from build123d import *

# Parameters (mm, degrees)
F2_R     = 1.5875
F3_DEPTH = 8.891
F4_SIZE  = 0.508
F5_SIZE  = 0.508


with BuildPart() as f1:
    # F0 (on Front) → F1 (revolve)
    with BuildSketch(Plane.XZ):
        Polygon((0.508, 6.35), (0, 6.35), (-0.508, 6.35), (-0.508, 10.16), (-2.0955, 10.16), (-4.445, 6.35), (-4.445, 0), (4.445, 0), (4.445, 6.35), (2.0955, 10.16), (0.508, 10.16), align=None)
    revolve(axis=Axis((0, 0, 0), (-1, 0, 0)))

    # F2 (on face) → F3 (cut, through all)
    with BuildSketch(Plane.YZ.offset(4.445)):
        Circle(F2_R)
    extrude(amount=-F3_DEPTH, mode=Mode.SUBTRACT)

    # F4
    f4_edges = [f1.edges().sort_by_distance(p)[0] for p in [
        (-4.445, -1.5875, 0),
        (4.445, -1.5875, 0),
    ]]
    chamfer(f4_edges, length=F4_SIZE)

    # F5
    f5_edges = [f1.edges().sort_by_distance(p)[0] for p in [
        (-0.508, 0, -10.16),
        (0.508, 0, -10.16),
    ]]
    chamfer(f5_edges, length=F5_SIZE)


solid = f1.part
Geometry: final body of the model. Coordinates: model frame, mm. A direction names the side the tool comes from. Coordinates: 2 decimals unless noted, no trailing zeros. Write each loop counter-clockwise with the first axis right and the second up, starting at its lowest first coordinate (ties: lowest second). Pieces come first, ordered by that corner, then holes. Notation, with made-up numbers: (65, 27) - (78, 27) arc R8 cw to (78, 36) - close; hole circle Ø10 at (60.25, 20). An arc over 180 degrees is marked (long way). Return JSON: item names as keys, results as strings.
Item 1: Pin query (flat end, axial travel): pin 1 Ø2.5 at (y, z) = (0, 0) entering from +X; pin 2 Ø1.5 at (x, y) = (-2, 4) entering from -Z; pin 3 Ø5 at (x, z) = (2.5, -5) entering from +Y; pin 4 Ø1.5 at (x, y) = (0, -7) entering from -Z. Return the tip coordinate at first contact, or that it passes through.
Completed:
{"pin 1": "passes through", "pin 2": "stops at z = -9.63", "pin 3": "stops at y = 9.84", "pin 4": "stops at z = -7.22"}
Item 2: Pull-direction query (Z, two-part tool) for faces 3 (the face through (-1.563, 10.074, -1.323)), 4 (the face through (0.508, -6.3, 2)), 5 (the face through (0.06, -0.34, -1.55)); classes: +Z half, -Z half, draft (parallel to the pull), parting line (faces both ways), or undercut.
Completed:
{"face 3": "parting line", "face 4": "draft", "face 5": "undercut"}
Item 3: Section query C-C (x = 1.75). Output: boundary loops of the cut face in (y, z) (1 decimal).
Completed:
{"outline": "circle Ø20.3 at (0, 0); hole circle Ø3.2 at (0, 0)"}
Item 4: Line query: L1, parallel to X at y = -9, z = 1.25; L2, parallel to X at y = 6.75, z = -7.25; L3, parallel to Z at x = -3.5, y = 1. Output: solid intervals per line, ascending.
Completed:
{"L1": "x = -2.76 to -0.51, 0.51 to 2.76", "L2": "x = -2.25 to -0.76, 0.76 to 2.25", "L3": "z = -7.82 to -1.23, 1.23 to 7.82"}
Item 5: Reachability of faces 1 (the face through (-0.01, -6.2, -1.38)), 2 (the face through (4.445, 2, 2)) from +Z, -Z, +X, -X, +Y, -Y: full face, straight path, thin tool, end or side. Return the list, or none.
Completed:
{"face 1": "none", "face 2": "+Z, -Z, +X, +Y, -Y"}
